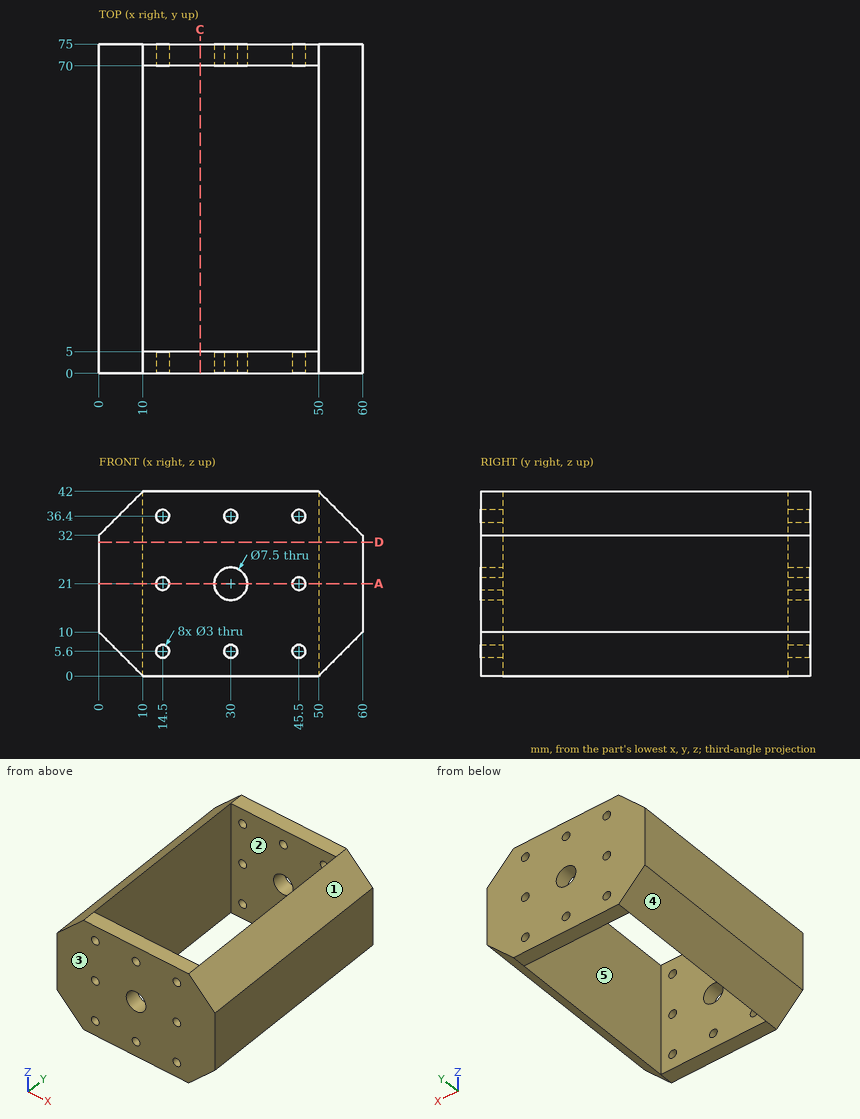
Design review of the part shown in the three views and the two pictorial views. Dimensions are in mm from the part's minimum x, y and z. A direction names the side the tool comes from. Round coordinates to 2 decimals unless told otherwise and drop trailing zeros. Loops run counter-clockwise (first coordinate to the right, second up) from the corner with the lowest first, then second, coordinate; pieces in that order, holes last.
1) Consider section C-C on x = 23. State the section outline as (y, z) points.
Values follow:
outline: (0, 0) - (5, 0) - (5, 42) - (0, 42) - close; (70, 0) - (75, 0) - (75, 42) - (70, 42) - close
2) Consider section D-D on z = 30.5. State the section outline as (x, y) points.
Values follow:
outline: (0, 0) - (60, 0) - (60, 75) - (0, 75) - close; hole (10, 5) - (50, 5) - (50, 70) - (10, 70) - close
3) Tool access review of the marked faces 4 and 5: name each direction out of +Z, -Z, +X, -X, +Y, -Y from which nothing blocks a thin tool from reaching the whole face with its end or side.
Values follow:
face 4: -Z, -X, +Y, -Y
face 5: +Z, -Z
4) Wall thickness on line 1 along Z through (x, y) = (45.5, 1.45); line 2 along X through (y, z) = (62, 30.5); line 3 along Y through (x, z) = (39.5, 15): over which ranges is each line inside the solid? List them lowest first.
Values follow:
line 1: z = 0 to 4.1, 7.1 to 19.5, 22.5 to 34.9, 37.9 to 42
line 2: x = 0 to 10, 50 to 60
line 3: y = 0 to 5, 70 to 75
5) Clearance check with a flat-ended pin moving along its axis: P1, Ø4, axis at x = 45.5, z = 36.4, coming from the -Y side. State where the tip first meets the part, or that it passes through.
Values follow:
P1: stops at y = 0
6) The part is to be moulded in two halves that separate along Y. For the marked faces 1, 2 and 3, say which applies: pulls with the +Y half, pulls with the -Y half, needs draft (parallel to the pull), parting line crosses it, or undercut.
Values follow:
face 1: needs draft
face 2: undercut
face 3: pulls with the -Y half
7) Consider section A-A on z = 21. Give the number of separate pieces and of enclosed holes in the cut face, then the cut area to 4 significant figures.
Values follow:
separate pieces: 6
enclosed holes: 0
area: 1,765 mm2
